Source: CAD feature listing. Evaluate the final solid. Frame: model axes, mm. Face numbers are marked on the shaded views. A direction names the side the tool comes from. Give positions to 0.01 mm unless a question says otherwise; leave off trailing zeros. Loops run counter-clockwise (first coordinate to the right, second up) from the corner with the lowest first, then second, coordinate; pieces in that order, holes last. Notation, with made-up numbers: M 31.5,-31 L 40.5,-31 A16 ccw 40.5,-22 Z; hole C 62.5,46.5 d4. An arc over 180 degrees is marked long. Answer in a Markdown table with one row per item.
```python
from build123d import *

# Parameters (mm, degrees)
SKETCH_1_W          = 55
SKETCH_1_H          = 20
EXTRUDE_1_DEPTH     = 2
SKETCH_3_W          = 1.5
SKETCH_3_H          = 20
EXTRUDE_2_DEPTH     = 35
FILLET_1_R          = 10
FILLET_3_R          = 1
CUT_EXTRUDE_1_REACH = 49.173
SKETCH_6_R          = 2.5
SKETCH_6_R_2        = 1


with BuildPart() as part:
    # 草图1 → 凸台-拉伸1 (new body)
    with BuildSketch(Plane(origin=(0, 0, 0), x_dir=(1, 0, 0), z_dir=(0, 1, 0))):
        Rectangle(SKETCH_1_W, SKETCH_1_H)
    extrude(amount=-EXTRUDE_1_DEPTH)

    # 草图3 → 凸台-拉伸2 (add)
    with BuildSketch(Plane(origin=(0, 0, 0), x_dir=(1, 0, 0), z_dir=(0, 1, 0))):
        with Locations((-26.75, 0)):
            Rectangle(SKETCH_3_W, SKETCH_3_H)
        with Locations((26.75, 0)):
            Rectangle(SKETCH_3_W, SKETCH_3_H)
    extrude(amount=EXTRUDE_2_DEPTH)

    # 圆角1
    fillet_1_edges = [part.edges().sort_by_distance(p)[0] for p in [
        (-26.75, 35, -10),
        (-26.75, 35, 10),
        (26.75, 35, 10),
        (26.75, 35, -10),
    ]]
    fillet(fillet_1_edges, radius=FILLET_1_R - 0.0001)  # a hair under: the kernel refuses the full size

    # 圆角3
    fillet_3_edges = [part.edges().sort_by_distance(p)[0] for p in [
        (-26, 0, 0),
        (26, 0, 0),
    ]]
    fillet(fillet_3_edges, radius=FILLET_3_R)

    # 草图6 → 切除-拉伸1 (cut, up to next)
    with BuildSketch(Plane.XZ.offset(2), mode=Mode.PRIVATE) as cut_extrude_1_sk1:
        with Locations(Location((0, 0, 0), (0, 0, 270))):
            Circle(SKETCH_6_R)
    cut_extrude_1_tool1 = extrude(cut_extrude_1_sk1.sketch, amount=-CUT_EXTRUDE_1_REACH, mode=Mode.PRIVATE) & part.part
    # 草图6 → 切除-拉伸1 (cut, up to next)
    with BuildSketch(Plane.XZ.offset(2), mode=Mode.PRIVATE) as cut_extrude_1_sk2:
        with Locations(Location((-5, 5, 0), (0, 0, 270))):
            Circle(SKETCH_6_R_2)
    cut_extrude_1_tool2 = extrude(cut_extrude_1_sk2.sketch, amount=-CUT_EXTRUDE_1_REACH, mode=Mode.PRIVATE) & part.part
    # 草图6 → 切除-拉伸1 (cut, up to next)
    with BuildSketch(Plane.XZ.offset(2), mode=Mode.PRIVATE) as cut_extrude_1_sk3:
        with Locations(Location((-5, -5, 0), (0, 0, 270))):
            Circle(SKETCH_6_R_2)
    cut_extrude_1_tool3 = extrude(cut_extrude_1_sk3.sketch, amount=-CUT_EXTRUDE_1_REACH, mode=Mode.PRIVATE) & part.part
    # 草图6 → 切除-拉伸1 (cut, up to next)
    with BuildSketch(Plane.XZ.offset(2), mode=Mode.PRIVATE) as cut_extrude_1_sk4:
        with Locations(Location((5, -5, 0), (0, 0, 270))):
            Circle(SKETCH_6_R_2)
    cut_extrude_1_tool4 = extrude(cut_extrude_1_sk4.sketch, amount=-CUT_EXTRUDE_1_REACH, mode=Mode.PRIVATE) & part.part
    # 草图6 → 切除-拉伸1 (cut, up to next)
    with BuildSketch(Plane.XZ.offset(2), mode=Mode.PRIVATE) as cut_extrude_1_sk5:
        with Locations(Location((5, 5, 0), (0, 0, 270))):
            Circle(SKETCH_6_R_2)
    cut_extrude_1_tool5 = extrude(cut_extrude_1_sk5.sketch, amount=-CUT_EXTRUDE_1_REACH, mode=Mode.PRIVATE) & part.part
    # 草图6 → 切除-拉伸1 (cut, up to next)
    with BuildSketch(Plane.XZ.offset(2), mode=Mode.PRIVATE) as cut_extrude_1_sk6:
        with Locations(Location((15, 5, 0), (0, 0, 270))):
            Circle(SKETCH_6_R_2)
    cut_extrude_1_tool6 = extrude(cut_extrude_1_sk6.sketch, amount=-CUT_EXTRUDE_1_REACH, mode=Mode.PRIVATE) & part.part
    # 草图6 → 切除-拉伸1 (cut, up to next)
    with BuildSketch(Plane.XZ.offset(2), mode=Mode.PRIVATE) as cut_extrude_1_sk7:
        with Locations(Location((-15, 5, 0), (0, 0, 90))):
            Circle(SKETCH_6_R_2)
    cut_extrude_1_tool7 = extrude(cut_extrude_1_sk7.sketch, amount=-CUT_EXTRUDE_1_REACH, mode=Mode.PRIVATE) & part.part
    # 草图6 → 切除-拉伸1 (cut, up to next)
    with BuildSketch(Plane.XZ.offset(2), mode=Mode.PRIVATE) as cut_extrude_1_sk8:
        with Locations(Location((15, -5, 0), (0, 0, 90))):
            Circle(SKETCH_6_R_2)
    cut_extrude_1_tool8 = extrude(cut_extrude_1_sk8.sketch, amount=-CUT_EXTRUDE_1_REACH, mode=Mode.PRIVATE) & part.part
    # 草图6 → 切除-拉伸1 (cut, up to next)
    with BuildSketch(Plane.XZ.offset(2), mode=Mode.PRIVATE) as cut_extrude_1_sk9:
        with Locations(Location((-15, -5, 0), (0, 0, 270))):
            Circle(SKETCH_6_R_2)
    cut_extrude_1_tool9 = extrude(cut_extrude_1_sk9.sketch, amount=-CUT_EXTRUDE_1_REACH, mode=Mode.PRIVATE) & part.part
    add(cut_extrude_1_tool1.solids().sort_by_distance((0, -2, 0))[0], mode=Mode.SUBTRACT)
    add(cut_extrude_1_tool2.solids().sort_by_distance((-5, -2, 5))[0], mode=Mode.SUBTRACT)
    add(cut_extrude_1_tool3.solids().sort_by_distance((-5, -2, -5))[0], mode=Mode.SUBTRACT)
    add(cut_extrude_1_tool4.solids().sort_by_distance((5, -2, -5))[0], mode=Mode.SUBTRACT)
    add(cut_extrude_1_tool5.solids().sort_by_distance((5, -2, 5))[0], mode=Mode.SUBTRACT)
    add(cut_extrude_1_tool6.solids().sort_by_distance((15, -2, 5))[0], mode=Mode.SUBTRACT)
    add(cut_extrude_1_tool7.solids().sort_by_distance((-15, -2, 5))[0], mode=Mode.SUBTRACT)
    add(cut_extrude_1_tool8.solids().sort_by_distance((15, -2, -5))[0], mode=Mode.SUBTRACT)
    add(cut_extrude_1_tool9.solids().sort_by_distance((-15, -2, -5))[0], mode=Mode.SUBTRACT)


solid = part.part
```
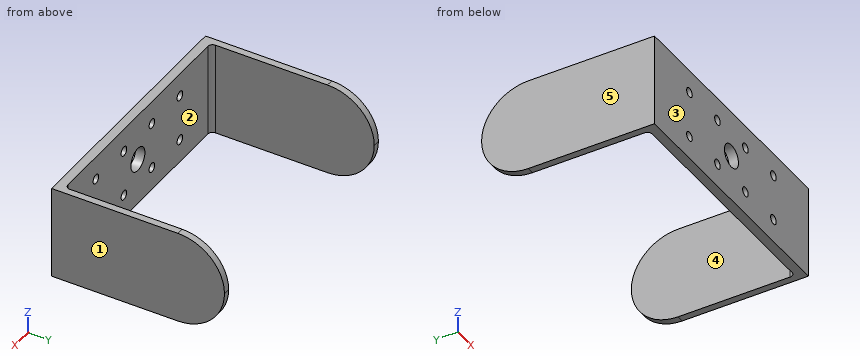
1) Section D-D, the plane z = 5. Return loops of the section in (x, y).
Reply:
| item | result |
|---|---|
| outline | M -27.5,-2 L -16,-2 L -16,0 L -25,0 A1 cw -26,1 L -26,33.66 L -27.5,33.66 Z; M -14,-2 L -6,-2 L -6,0 L -14,0 Z; M -4,-2 L 4,-2 L 4,0 L -4,0 Z; M 6,-2 L 14,-2 L 14,0 L 6,0 Z; M 16,-2 L 27.5,-2 L 27.5,33.66 L 26,33.66 L 26,1 A1 cw 25,0 L 16,0 Z |
2) Section A-A, the plane y = 5.5. Return loops of the section in (x, z), then the cut area to 3 significant figures.
Reply:
| item | result |
|---|---|
| outline | M -27.5,-10 L -26,-10 L -26,10 L -27.5,10 Z; M 26,-10 L 27.5,-10 L 27.5,10 L 26,10 Z |
| area | 60.0 mm² |
3) Set-up query: the marked faces 1 and 2. Return all of +Z, -Z, +X, -X, +Y, -Y with unobstructed straight access to the full face (end or side cutting, diameter ignored); none if empty.
Reply:
| item | result |
|---|---|
| face 1 | +Z, -Z, +X, +Y, -Y |
| face 2 | +Z, -Z, +Y |
4) Section C-C, the plane z = -1.25. Return loops of the section in (x, y), then the cut area to 3 significant figures.
Reply:
| item | result |
|---|---|
| outline | M -27.5,-2 L -2.17,-2 L -2.17,0 L -25,0 A1 cw -26,1 L -26,34.92 L -27.5,34.92 Z; M 2.17,-2 L 27.5,-2 L 27.5,34.92 L 26,34.92 L 26,1 A1 cw 25,0 L 2.17,0 Z |
| area | 207 mm² |
5) Pin query (flat end, axial travel): pin 1 Ø2.5 at (x, z) = (-15, 5) entering from +Y. Return the tip coordinate at first contact, or that it passes through.
Reply:
| item | result |
|---|---|
| pin 1 | stops at y = 0 |
6) Material intervals for L1, parallel to X at y = -1.15, z = 5; L2, parallel to X at y = 29, z = 7.75; L3, parallel to Y at x = 21, z = 4.25, sorted ascending.
Reply:
| item | result |
|---|---|
| L1 | x = -27.5 to -16, -14 to -6, -4 to 4, 6 to 14, 16 to 27.5 |
| L2 | x = -27.5 to -26, 26 to 27.5 |
| L3 | y = -2 to 0 |
7) Pull-direction query (X, two-part tool) for the marked faces 3, 4 and 5; classes: released by +X, released by -X, zero draft, split by the parting line, or undercut.
Reply:
| item | result |
|---|---|
| face 3 | zero draft |
| face 4 | undercut |
| face 5 | released by -X |
8) Section B-B, the plane x = 5. Return loops of the section in (y, z).
Reply:
| item | result |
|---|---|
| outline | M -2,-10 L 0,-10 L 0,-6 L -2,-6 Z; M -2,-4 L 0,-4 L 0,4 L -2,4 Z; M -2,6 L 0,6 L 0,10 L -2,10 Z |
